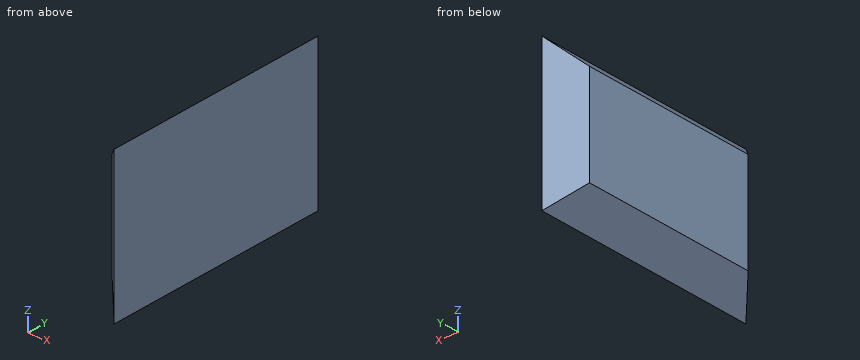
Autodesk Inventor part; units mm, degrees
ref_plane "YZ Plane" through (0, 0, 0) normal (1, 0, 0) x (0, 1, 0)
ref_plane "XZ Plane" through (0, 0, 0) normal (0, 1, 0) x (-1, 0, 0)
ref_plane "XY Plane" through (0, 0, 0) normal (0, 0, 1) x (1, 0, 0)
sketch "Sketch1" plane through (0, 0, 0) normal (1, 0, 0) x (0, 1, 0)
  line L0 (0, 0) -> (90, 0)
  line L1 (90, 0) -> (90, 60)
  line L2 (90, 60) -> (0, 60)
  line L3 (0, 60) -> (0, 0)
  dimension "d0" = 90
  dimension "d1" = 60
extrude "Extrusion1" add sketch "Sketch1" along normal blind 10
chamfer "Chamfer1" distance 10 angle 45 1 edges at (0, 0, 30)
chamfer "Chamfer2" distance 10 angle 45 1 edges at (0, 49.9997, 60)
chamfer "Chamfer3" distance 10 angle 45 1 edges at (0, 90, 25.0003)
chamfer "Chamfer4" distance 10 angle 45 1 edges at (0, 45, 0)
properties part number "pied"
Model file for the job. Use its own axes, mm. Coordinates: 2 decimals unless noted, no trailing zeros. Loops run counter-clockwise (first coordinate to the right, second up) from the corner with the lowest first, then second, coordinate; pieces in that order, holes last. Notation, with made-up numbers: M 53,61.5 L 110,61.5 A25 ccw 110,74.5 Z; hole C 13,53.5 d2. An arc over 180 degrees is marked long. Use CSV: the item, a comma, the result in double quotes. Start each with the question number.
1. Flat gauge pins, fed straight in: pin 1 (1.5 mm diameter, centred on x = 3, y = 22.5, fed in from -Z); pin 2 (5 mm diameter, centred on x = 6.5, z = 53.5, fed in from +Y); pin 3 (1.5 mm diameter, centred on x = 4.5, z = 22.5, fed in from -Y). Where does each tip first touch, or does it go through?
2. Band-saw the part on D-D, the plane x = 6.5. List the corners of the cut face in (y, z).
3. Probe probe 1 along Y at (x, z) = (4.5, 49); probe 2 along Y at (x, z) = (5.25, 26.5); probe 3 along Z at (x, y) = (6.5, 51.5). List the from-to ranges inside material, lowest first. Write a range as [from, to].
4. Band-saw the part on C-C, the plane x = 2. List the corners of the cut face in (y, z).
Entries:
1,pin 1,"stops at z = 6.25"
1,pin 2,"stops at y = 89"
1,pin 3,"stops at y = 4.75"
2,outline,"M 3.5,3.5 L 86.5,3.5 L 86.5,56.5 L 3.5,56.5 Z"
3,probe 1,"y = [5.5, 84.5]"
3,probe 2,"y = [4.75, 85.25]"
3,probe 3,"z = [3.5, 56.5]"
4,outline,"M 8,8 L 82,8 L 82,52 L 8,52 Z"
